For this review, take the finished solid that the model builds, in its own axes (mm). Coordinates: 2 decimals unless noted, no trailing zeros. Order: outer loops, then holes, each group sorted by start corner. A loop starts at its lowest first (then second) coordinate and runs counter-clockwise, first axis right, second up. Notation, with made-up numbers: (69, 17) -> (100, 17) arc R5 cw to (100, 26) -> close; hole circle Ø2 at (25.5, 7). An arc over 180 degrees is marked (long way). Answer as a JSON object with one key per item and string values. Group by question number.
1) Add section B-B, the plane y = 1. Write out the cut boundary in (x, z), then the cut area to 3 significant figures.
2) Wall thickness on L1, parallel to X at y = 1.6, z = -27; L2, parallel to X at y = 0.6, z = 242; L3, parallel to Y at x = 1.5, z = -206.5: over which ranges is each line inside the solid? List them lowest first.
3) Add section C-C, the plane x = 0.5. Write out the cut boundary in (y, z).
4) Add section A-A, the plane z = -226.5. Write out the cut boundary in (x, y).
5) For pin 1 (1.7 mm diameter, centred on x = -0.5, z = 28.5, fed in from -Y), flat-tipped, find the tip position at first contact; note if it passes through.
from build123d import *

# Parameters (mm, degrees)
BOSS_EXTRUDE1_DEPTH = 266.75


with BuildPart() as part:
    # Sketch1 → Boss-Extrude1 (new body, symmetric)
    with BuildSketch(Plane.XY):
        with BuildLine():
            Line((-3.6, 3.35), (-3, 0))
            Line((-3, 0), (-2.2, 0))
            Line((-2.2, 0), (-2.735217071, 2.988295315))
            ThreePointArc((-2.735217071, 2.988295315), (-2.659117427, 3.274614514), (-2.390699246, 3.4))
            Line((-2.390699246, 3.4), (-2.2, 3.4))
            Line((-2.2, 3.4), (-2.070472639, 4.88050451))
            ThreePointArc((-2.070472639, 4.88050451), (-1.958261067, 5.108047068), (-1.721804495, 5.2))
            Line((-1.721804495, 5.2), (1.721804495, 5.2))
            ThreePointArc((1.721804495, 5.2), (1.958261067, 5.108047068), (2.070472639, 4.88050451))
            Line((2.070472639, 4.88050451), (2.2, 3.4))
            Line((2.2, 3.4), (2.390699246, 3.4))
            ThreePointArc((2.390699246, 3.4), (2.659117427, 3.274614514), (2.735217071, 2.988295315))
            Line((2.735217071, 2.988295315), (2.2, 0))
            Line((2.2, 0), (3, 0))
            Line((3, 0), (3.6, 3.35))
            ThreePointArc((3.6, 3.35), (3.497487373, 3.597487373), (3.25, 3.7))
            Line((3.25, 3.7), (3, 3.7))
            Line((3, 3.7), (2.835477174, 5.58050451))
            ThreePointArc((2.835477174, 5.58050451), (2.723265602, 5.808047068), (2.486809029, 5.9))
            Line((2.486809029, 5.9), (-2.486809029, 5.9))
            ThreePointArc((-2.486809029, 5.9), (-2.723265602, 5.808047068), (-2.835477174, 5.58050451))
            Line((-2.835477174, 5.58050451), (-3, 3.7))
            Line((-3, 3.7), (-3.25, 3.7))
            ThreePointArc((-3.25, 3.7), (-3.497487373, 3.597487373), (-3.6, 3.35))
        make_face()
    extrude(amount=BOSS_EXTRUDE1_DEPTH, both=True)


solid = part.part
Output values:
{
 "1": {"outline": "(-3.18, -266.75) -> (-2.38, -266.75) -> (-2.38, 266.75) -> (-3.18, 266.75) -> close; (2.38, -266.75) -> (3.18, -266.75) -> (3.18, 266.75) -> (2.38, 266.75) -> close", "area": "854 mm²"},
 "2": {"L1": "x = -3.29 to -2.49, 2.49 to 3.29", "L2": "x = -3.11 to -2.31, 2.31 to 3.11", "L3": "y = 5.2 to 5.9"},
 "3": {"outline": "(5.2, -266.75) -> (5.9, -266.75) -> (5.9, 266.75) -> (5.2, 266.75) -> close"},
 "4": {"outline": "(-3.6, 3.35) -> (-3, 0) -> (-2.2, 0) -> (-2.74, 2.99) arc R0.35 cw to (-2.39, 3.4) -> (-2.2, 3.4) -> (-2.07, 4.88) arc R0.35 cw to (-1.72, 5.2) -> (1.72, 5.2) arc R0.35 cw to (2.07, 4.88) -> (2.2, 3.4) -> (2.39, 3.4) arc R0.35 cw to (2.74, 2.99) -> (2.2, 0) -> (3, 0) -> (3.6, 3.35) arc R0.35 ccw to (3.25, 3.7) -> (3, 3.7) -> (2.84, 5.58) arc R0.35 ccw to (2.49, 5.9) -> (-2.49, 5.9) arc R0.35 ccw to (-2.84, 5.58) -> (-3, 3.7) -> (-3.25, 3.7) arc R0.35 ccw to start"},
 "5": {"pin 1": "stops at y = 5.2"}
}
